```python
from build123d import *

# Parameters (mm, degrees)
CROQUIS1_R              = 3.75
CROQUIS1_R_2            = 1.249999997
CROQUIS1_R_3            = 1.25
CROQUIS1_R_4            = 1.250000007
CROQUIS1_R_5            = 1.6
SALIENTE_EXTRUIR1_DEPTH = 1.6


with BuildPart() as part:
    # Croquis1 → Saliente-Extruir1 (new body)
    with BuildSketch(Plane.XY):
        with BuildLine():
            Line((-17.5, -10.1), (17.5, -10.1))
            Line((17.5, -10.1), (17.5, -3.744033218))
            ThreePointArc((17.5, -3.744033218), (17.210606187, -2.056801008), (16.375506293, -0.562441789))
            Line((16.375506293, -0.562441789), (6.757496482, 7.466348016))
            ThreePointArc((6.757496482, 7.466348016), (0, 10.070258755), (-6.757496482, 7.466348016))
            Line((-6.757496482, 7.466348016), (-16.375506293, -0.562441789))
            ThreePointArc((-16.375506293, -0.562441789), (-17.210606187, -2.056801008), (-17.5, -3.744033218))
            Line((-17.5, -3.744033218), (-17.5, -10.1))
        make_face()
        Circle(CROQUIS1_R, mode=Mode.SUBTRACT)
        with Locations((-0.0012, 5.99880001)):
            Circle(CROQUIS1_R_2, mode=Mode.SUBTRACT)
        with Locations((5.194513192, 3.000439231)):
            Circle(CROQUIS1_R_3, mode=Mode.SUBTRACT)
        with Locations((5.195713192, -2.998360769)):
            Circle(CROQUIS1_R_3, mode=Mode.SUBTRACT)
        with Locations((0.0012, -5.9988)):
            Circle(CROQUIS1_R_3, mode=Mode.SUBTRACT)
        with Locations((-5.194513192, -3.00043923)):
            Circle(CROQUIS1_R_3, mode=Mode.SUBTRACT)
        with Locations((-5.195713248, 2.998360802)):
            Circle(CROQUIS1_R_4, mode=Mode.SUBTRACT)
        with Locations((12.3, -4.3)):
            Circle(CROQUIS1_R_5, mode=Mode.SUBTRACT)
        with Locations((-12.3, -4.3)):
            Circle(CROQUIS1_R_5, mode=Mode.SUBTRACT)
    extrude(amount=SALIENTE_EXTRUIR1_DEPTH)


solid = part.part
```
CAD build for the part. Positions are in the model's coordinates, mm. Coordinates: 2 decimals unless noted, no trailing zeros. Loops run counter-clockwise (first coordinate to the right, second up) from the corner with the lowest first, then second, coordinate; pieces in that order, holes last. Notation, with made-up numbers: (-32, 65.25) - (-14, 65.25) arc R9 ccw to (-14, 72.25) - close; hole circle Ø10 at (29, 69). An arc over 180 degrees is marked (long way). Return JSON: item names as keys, results as strings.
1. Band-saw the part on A-A (x = 0). Give the cut face in (y, z).
Result:
{"outline": "(-10.1, 0) - (-7.25, 0) - (-7.25, 1.6) - (-10.1, 1.6) - close; (-4.75, 0) - (-3.75, 0) - (-3.75, 1.6) - (-4.75, 1.6) - close; (3.75, 0) - (4.75, 0) - (4.75, 1.6) - (3.75, 1.6) - close; (7.25, 0) - (10.07, 0) - (10.07, 1.6) - (7.25, 1.6) - close"}
2. Mould opens along Y. For faces 1 (the flat face through (0, -4, 0)), 2 (the cylindrical face through (6.35, -3.48, 0.79)), 3 (the flat face through (-11.5, 3.51, 0.79)) say: released by +Y, released by -Y, zero draft, split by the parting line, or undercut.
Result:
{"face 1": "zero draft", "face 2": "undercut", "face 3": "released by +Y"}
3. Band-saw the part on B-B (y = 0). Give the cut face in (x, z).
Result:
{"outline": "(-15.7, 0) - (-3.75, 0) - (-3.75, 1.6) - (-15.7, 1.6) - close; (3.75, 0) - (15.7, 0) - (15.7, 1.6) - (3.75, 1.6) - close"}
4. Probe L1, parallel to X at y = 2.75, z = 0.65; L2, parallel to Y at x = -5, z = 1.45; L3, parallel to X at y = 4, z = 0.5. List the from-to ranges inside material, lowest first. Write a range as from..to.
Result:
{"L1": "x = -12.41..-6.42, -3.97..-2.55, 2.55..3.97, 6.42..12.41", "L2": "y = -10.1..-4.24, -1.77..1.76, 4.23..8.74", "L3": "x = -10.91..-5.94, -4.45..4.44, 5.95..10.91"}
5. Band-saw the part on D-D (z = 1). State how many separate pieces and enclosed holes the cut face has, and give its area (3 significant figures).
Result:
{"separate pieces": "1", "enclosed holes": "9", "area": "452 mm2"}
6. Band-saw the part on C-C (x = 11.5). Give the cut face in (y, z), and give its area (3 significant figures).
Result:
{"outline": "(-10.1, 0) - (-5.69, 0) - (-5.69, 1.6) - (-10.1, 1.6) - close; (-2.91, 0) - (3.51, 0) - (3.51, 1.6) - (-2.91, 1.6) - close", "area": "17.3 mm2"}
